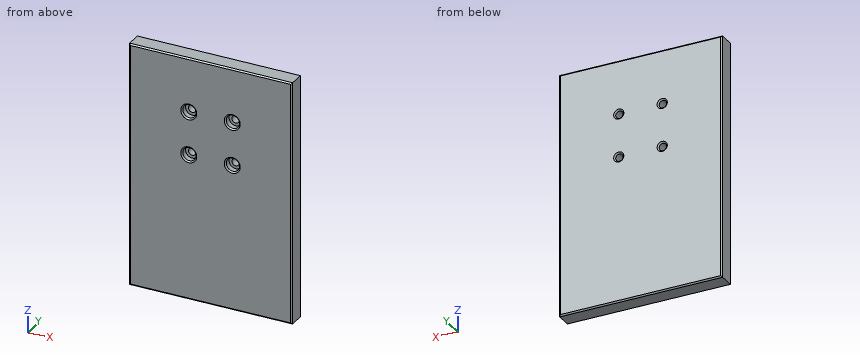
```python
from build123d import *

# Parameters (mm, degrees)
F0_W           = 120
F0_H           = 180
F1_DEPTH       = 13
F3_D           = 5.5
F3_CBORE_D     = 9.75
F3_CBORE_DEPTH = 5
F4_SIZE        = 1
F5_SIZE        = 1


with BuildPart() as f1:
    # F0 (on Front) → F1 (new body)
    with BuildSketch(Plane.XZ):
        with Locations((60, 90)):
            Rectangle(F0_W, F0_H)
    extrude(amount=F1_DEPTH)

    # F3 (through all)
    with Locations(Plane.XZ.offset(13)):
        with Locations((44, 140), (44, 108), (76, 140), (76, 108)):
            CounterBoreHole(F3_D / 2, F3_CBORE_D / 2, F3_CBORE_DEPTH)

    # F4
    f4_edges = [f1.edges().sort_by_distance(p)[0] for p in [
        (60, -13, 180),
        (0, -13, 90),
        (60, -13, 0),
        (120, -13, 90),
        (39.125, -13, 108),
        (71.125, -13, 108),
        (39.125, -13, 140),
        (71.125, -13, 140),
    ]]
    chamfer(f4_edges, length=F4_SIZE)

    # F5
    f5_edges = [f1.edges().sort_by_distance(p)[0] for p in [
        (0, 0, 90),
        (60, 0, 180),
        (60, 0, 0),
        (120, 0, 90),
        (41.25, 0, 108),
        (73.25, 0, 108),
        (41.25, 0, 140),
        (73.25, 0, 140),
    ]]
    chamfer(f5_edges, length=F5_SIZE)


solid = f1.part
```
Geometry check sheet. Reference: the model listing, model coordinates, mm. Coordinates: 2 decimals unless noted, no trailing zeros. One line per item, written item: value. Start each with the question number.
(1) Depth check by flat-ended pin: pin 1 (15.5 mm diameter, centred on x = 76, z = 140, fed in from +Y); pin 2 (3 mm diameter, centred on x = 45.5, z = 109.5, fed in from -Y); pin 3 (6.5 mm diameter, centred on x = 76, z = 140, fed in from +Y). Enter the tip coordinate at first touch or a pass-through.
(2) Sectioned sample at A-A, the plane z = 108. State how many separate pieces and enclosed holes the cut face has, and give its area (3 significant figures).
(3) Scan lines: line 1 along Z through (x, y) = (44, -4.75); line 2 along X through (y, z) = (-6, 140); line 3 along Z through (x, y) = (76, -10.3) (3 decimals). Record each from-to range of solid material in increasing order. Write a range as [from, to].
Filled sheet:
1. pin 1: y = 0
1. pin 2: y = -8
1. pin 3: y = -0.5
2. separate pieces: 3
2. enclosed holes: 0
2. area: 1,370 mm²
3. line 1: [0, 105.25], [110.75, 137.25], [142.75, 180]
3. line 2: [0, 41.25], [46.75, 73.25], [78.75, 120]
3. line 3: [0, 103.125], [112.875, 135.125], [144.875, 180]
